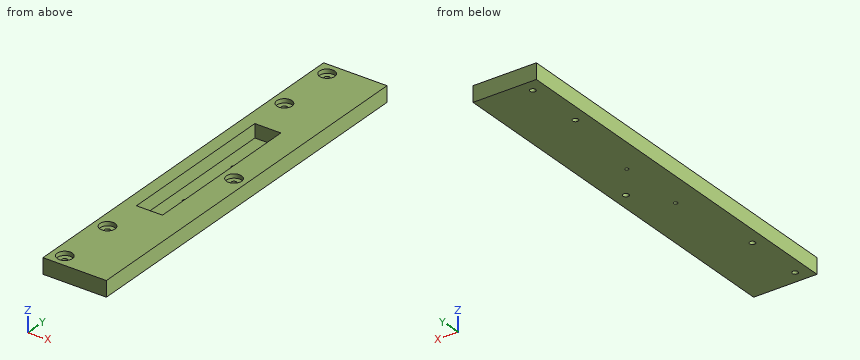
Autodesk Inventor part; units mm, degrees
ref_plane "YZ Plane" through (0, 0, 0) normal (1, 0, 0) x (0, 1, 0)
ref_plane "XZ Plane" through (0, 0, 0) normal (0, 1, 0) x (-1, 0, 0)
ref_plane "XY Plane" through (0, 0, 0) normal (0, 0, 1) x (1, 0, 0)
sketch "Sketch1" plane through (0, 0, 0) normal (0, 0, 1) x (1, 0, 0)
  line L0 (-30, 230) -> (45, 230)
  line L1 (45, 230) -> (45, -230)
  line L2 (45, -230) -> (-30, -230)
  line L3 (-30, -230) -> (-30, 230)
  point P0 (0, 0)
  dimension "d0" = 30
  dimension "d1" = 45
  dimension "d2" = 460
  dimension "d3" = 230
extrude "baseExtrusion" add sketch "Sketch1" along normal blind 2.5
sketch "Sketch2" plane through (0, 0, 2.5) normal (0, 0, 1) x (1, 0, 0)
  line L0 (-30, 230) -> (-30, -230)
  point P0 (0, 0)
  point P1 (0, 40)
  point P2 (0, -40)
  dimension "d6" = 80
  dimension "d7" = 40
  dimension "d8" = 30
  dimension "d9" = 30
hole "xyStageAttatchM5" at (0, 40, 2.5) at (0, -40, 2.5) direction (0, 0, -1) diameter 4.134 depth 14.2 tip angle 118
sketch "Sketch3" plane through (0, 0, 2.5) normal (0, 0, 1) x (1, 0, 0)
  line L0 (-30, 230) -> (45, 230)
  line L1 (45, 230) -> (45, -230)
  line L2 (45, -230) -> (-30, -230)
  line L3 (-30, -230) -> (-30, 230)
  line L4 (45, 230) -> (-30, 230)
  line L5 (-30, -230) -> (45, -230)
  line L6 (45, -230) -> (45, 230)
  line L7 (-30, 230) -> (-30, -230)
  line L8 (-15.3915, 97.0335) -> (15.3915, 97.0335)
  line L9 (15.3915, 97.0335) -> (15.3915, -97.0335)
  line L10 (15.3915, -97.0335) -> (-15.3915, -97.0335)
  line L11 (-15.3915, -97.0335) -> (-15.3915, 97.0335)
  point P0 (0, 0)
  dimension "d17" = 194.0669
  dimension "d18" = 97.0335
  dimension "d19" = 30.783
  dimension "d20" = 15.3915
extrude "Extrusion2" add sketch "Sketch3" along normal blind 16
sketch "Sketch4" plane through (0, 0, 18.5) normal (0, 0, 1) x (1, 0, 0)
  line L0 (-30, -230) -> (45, -230)
  line L1 (45, -230) -> (45, 230)
  line L2 (-30, 230) -> (-30, -230)
  point P0 (0, 0)
  point P1 (-15, -215)
  point P2 (-15, -145)
  point P3 (30, 0)
  dimension "d23" = 15
  dimension "d24" = 70
  dimension "d33" = 15
  dimension "d34" = 15
hole "Hole2" at (-15, -215, 18.5) at (-15, -145, 18.5) at (30, 0, 18.5) direction (0, 0, -1) diameter 6.6 end through all counterbore diameter 18 counterbore depth 4.8
mirror "Mirror1" about plane through (0, 0, 0) normal (0, 1, 0) of "Hole2"
properties part number "xyStageStilt"
Build history of the part. All positions in model axes, mm. Give positions to 0.01 mm unless a question says otherwise; leave off trailing zeros. Loops run counter-clockwise (first coordinate to the right, second up) from the corner with the lowest first, then second, coordinate; pieces in that order, holes last. Notation, with made-up numbers: (-33.5, 15.25) -> (19.5, 15.25) arc R26 ccw to (19.5, 36.25) -> close; hole circle Ø7 at (-25, -12). An arc over 180 degrees is marked (long way). Answer in a Markdown table with one row per item.
Item 1: Flat gauge pin, fed straight in: P1, Ø5.5, axis at x = 32.5, y = 4, coming from the +Z side. Where does the tip first touch, or does it go through?
Findings below:
| item | result |
|---|---|
| P1 | stops at z = 13.7 |
Item 2: Probe line 1 along Y through (x, z) = (-15, 10.75); line 2 along X through (y, z) = (0, 16.85); line 3 along X through (y, z) = (-40, 1.1). List the from-to ranges inside material, lowest first. Write a range as [from, to].
Findings below:
| item | result |
|---|---|
| line 1 | y = [-230, -218.3], [-211.7, -148.3], [-141.7, -97.03], [97.03, 141.7], [148.3, 211.7], [218.3, 230] |
| line 2 | x = [-30, -15.39], [15.39, 21], [39, 45] |
| line 3 | x = [-30, -2.07], [2.07, 45] |
Item 3: Slice it at A-A on y = -33.5. Write the cut outline in (x, z).
Findings below:
| item | result |
|---|---|
| outline | (-30, 0) -> (45, 0) -> (45, 18.5) -> (15.39, 18.5) -> (15.39, 2.5) -> (-15.39, 2.5) -> (-15.39, 18.5) -> (-30, 18.5) -> close |
Item 4: Slice it at B-B on x = 11.5. Write the cut outline in (y, z), plus the area to 3 significant figures.
Findings below:
| item | result |
|---|---|
| outline | (-230, 0) -> (230, 0) -> (230, 18.5) -> (97.03, 18.5) -> (97.03, 2.5) -> (-97.03, 2.5) -> (-97.03, 18.5) -> (-230, 18.5) -> close |
| area | 5,400 mm² |
